```python
from build123d import *

# Parameters (mm, degrees)
F0_W          = 30
F0_H          = 55
F1_DEPTH      = 1.5
F2_W          = 1.5
F2_H          = 55
F3_DEPTH      = 1.5
F3_DEPTH_BACK = 8
F4_DEPTH      = 28
F5_R          = 1
F6_DEPTH      = 1.5


with BuildPart() as f1:
    # F0 (on Top) → F1 (new body)
    with BuildSketch(Plane.XY):
        Rectangle(F0_W, F0_H)
    extrude(amount=F1_DEPTH)

    # F2 (on Top) → F3 (join, two sides)
    with BuildSketch(Plane.XY) as f3_sk:
        with Locations((-15.75, 0)):
            Rectangle(F2_W, F2_H)
    extrude(amount=F3_DEPTH)
    extrude(f3_sk.sketch, amount=-F3_DEPTH_BACK)

    # F2 (on Top) → F4 (join)
    with BuildSketch(Plane.XY):
        with Locations((15.75, 0)):
            Rectangle(F2_W, F2_H)
    extrude(amount=F4_DEPTH)

    # F5 (on face) → F6 (cut, through all)
    with BuildSketch(Plane(origin=(-16.5, 0, 0), x_dir=(0, -1, 0), z_dir=(-1, 0, 0))):
        with Locations((-24.5, -3)):
            Circle(F5_R)
        with Locations((5.5, -3)):
            Circle(F5_R)
    extrude(amount=-F6_DEPTH, mode=Mode.SUBTRACT)

    # F7: F1 across face


with BuildPart() as f1_1:
    add(f1.part)
    add(f1.part.mirror(Plane(origin=(15.75, 0, 28), x_dir=(1, 0, 0), z_dir=(0, 0, 1))))


solid = f1_1.part
```
CAD build for the part. Positions are in the model's coordinates, mm. A direction names the side the tool comes from. Round coordinates to 2 decimals unless told otherwise and drop trailing zeros. Order: outer loops, then holes, each group sorted by start corner. A loop starts at its lowest first (then second) coordinate and runs counter-clockwise, first axis right, second up.
Q1. Slice it at D-D (y = 24.5). Write the cut outline in (x, z), and give its area (4 significant figures).
Q2. Slice it at B-B (x = 6). Write the cut outline in (y, z).
Q3. Slice it at A-A (z = 59). Write the cut outline in (x, y).
Q4. Slice it at C-C (y = -17.5). Write the cut outline in (x, z).
Q5. Two-plate mould, pull along Z, no slides. Class faces 4 (the cylindrical face through (-15.8, 25.5, -3)), 5 (the flat face through (-1, 0, 1.5)), 6 (the flat face through (-15, 0, 60)), 7 (the flat face through (1, 0, 56)): pulls with the +Z half, pulls with the -Z half, needs draft (parallel to the pull), parting line crosses it, or undercut.
Q6. Which spindle directions (+Z, -Z, +X, -X, +Y, -Y) get a long thin tool onto all of the face, cutting with end or side? Do faces 1 (the flat face through (-16, 0, 64)), 2 (the flat face through (1, 0, 0)), 3 (the flat face through (15, 0, 28)). Say none if no direction does.
Q7. Wall check: L1, parallel to Y at x = -15.45, z = 59; L2, parallel to Z at x = -15.75, y = 24.5; L3, parallel to Z at x = 11.5, y = 13. Give the ranges that are in metal, low to high.
Q8. Drop flat-ended pins along their axis: pin 1 (9.5 mm diameter, centred on x = -4, y = -0.5, fed in from -Z); pin 2 (4 mm diameter, centred on y = -2, z = 60, fed in from +X); pin 3 (5 mm diameter, centred on x = -5, y = 11, fed in from +Z). Give the stop position or say it passes through.
Results below:
1. outline: (-16.5, -8) - (-15, -8) - (-15, -4) - (-16.5, -4) - close; (-16.5, -2) - (-15, -2) - (-15, 0) - (16.5, 0) - (16.5, 56) - (-15, 56) - (-15, 58) - (-16.5, 58) - (-16.5, 54.5) - (15, 54.5) - (15, 1.5) - (-16.5, 1.5) - close; (-16.5, 60) - (-15, 60) - (-15, 64) - (-16.5, 64) - close
1. area: 196.5 mm2
2. outline: (-27.5, 0) - (27.5, 0) - (27.5, 1.5) - (-27.5, 1.5) - close; (-27.5, 54.5) - (27.5, 54.5) - (27.5, 56) - (-27.5, 56) - close
3. outline: (-16.5, -27.5) - (-15, -27.5) - (-15, -6.5) - (-16.5, -6.5) - close; (-16.5, -4.5) - (-15, -4.5) - (-15, 23.5) - (-16.5, 23.5) - close; (-16.5, 25.5) - (-15, 25.5) - (-15, 27.5) - (-16.5, 27.5) - close
4. outline: (-16.5, -8) - (-15, -8) - (-15, 0) - (16.5, 0) - (16.5, 56) - (-15, 56) - (-15, 64) - (-16.5, 64) - (-16.5, 54.5) - (15, 54.5) - (15, 1.5) - (-16.5, 1.5) - close
5. face 4: undercut
5. face 5: undercut
5. face 6: needs draft
5. face 7: pulls with the +Z half
6. face 1: +Z, +X, -X, +Y, -Y
6. face 2: -Z, +X, +Y, -Y
6. face 3: -X, +Y, -Y
7. L1: y = -27.5 to -6.5, -4.5 to 23.5, 25.5 to 27.5
7. L2: z = -8 to -4, -2 to 1.5, 54.5 to 58, 60 to 64
7. L3: z = 0 to 1.5, 54.5 to 56
8. pin 1: stops at z = 0
8. pin 2: stops at x = -15
8. pin 3: stops at z = 56
